Verification items for the finished model (mm, model axes). A direction names the side the tool comes from. Coordinates: 2 decimals unless noted, no trailing zeros. Loops run counter-clockwise (first coordinate to the right, second up) from the corner with the lowest first, then second, coordinate; pieces in that order, holes last. Notation, with made-up numbers: (36, 74) -> (61, 74) arc R31 ccw to (61, 103) -> close; hole circle Ø3 at (-22, 34). An arc over 180 degrees is marked (long way). Answer as a JSON object with one key per item and string values. Group by question number.
Q1. Gauge pin test, flat ends, axial feed: pin 1 Ø2 at (x, y) = (-21.5, -30.5) entering from -Z; pin 2 Ø1.1 at (x, y) = (-29.5, -30) entering from -Z; pin 3 Ø2 at (x, y) = (8, 35) entering from -Z; pin 4 Ø8 at (x, y) = (8.5, 27) entering from -Z. Record the tip position at first contact, or that the pin passes through.
Q2. Scan lines: L1, parallel to Y at x = 21.5, z = 6.25; L2, parallel to Y at x = 31, z = 4; L3, parallel to X at y = 31, z = 2. Record each from-to range of solid material in increasing order.
Q3. Cross-section at B-B on y = 10. Record the boundary of the cut face in (x, z).
Q4. Release check for a two-part mould opening along Y. For faces 1 (the flat face through (-30, 34.858, 8)), 2 (the flat face through (-26.56, -30.76, 11.35)), 3 (the flat face through (-28.03, 34.34, 1.48)) record: released by +Y, released by -Y, zero draft, split by the parting line, or undercut.
Q5. Set-up check for faces 4 (the flat face through (32, 2, 0)), 5 (the flat face through (-14.262, 34.872, 12.506)), 6 (the flat face through (-28.03, -28.22, 3.48)), 7 (the flat face through (4, 35, 5)), 8 (the flat face through (0, -31, 20)): record each of +Z, -Z, +X, -X, +Y, -Y from which the full face is reachable in a straight line by a thin tool's end or side.
Q6. Cross-section at C-C on x = 25.5. Record the boundary of the cut face in (y, z), and give its area (3 significant figures).
Q7. Cross-section at D-D on x = -30. Record the boundary of the cut face in (y, z), and give its area (3 significant figures).
Q8. Cross-section at A-A on z = 1. Record the boundary of the cut face in (x, y).
```python
from build123d import *

# Parameters (mm, degrees)
SKETCH2_W               = 70
SKETCH2_H               = 67.6
BOSS_EXTRUDE2_DEPTH     = 20
SKETCH3_W               = 49.211808989
SKETCH3_H               = 73.758147992
CUT_EXTRUDE1_DEPTH      = 5
SHELL1_T                = -2
CHAMFER1_SIZE           = 3
CHAMFER2_SIZE           = 3
CUT_EXTRUDE2_REACH      = 80.917
FILLET1_R               = 1
FILLET1_OF_MIRROR1_R    = 1
SKETCH6_W               = 4.489342342
SKETCH6_H               = 3.232194467
CUT_EXTRUDE3_DEPTH      = 1
MIRROR3_COPY_1_SKETCH_W = 4.489342342
MIRROR3_COPY_1_SKETCH_H = 3.232194467
MIRROR3_COPY_1_DEPTH    = 1


with BuildPart() as part:
    # Sketch2 → Boss-Extrude2 (new body)
    with BuildSketch(Plane.XY):
        with Locations((0.470659816, 2.057998975)):
            Rectangle(SKETCH2_W, SKETCH2_H)
    extrude(amount=BOSS_EXTRUDE2_DEPTH)

    # Sketch3 → Cut-Extrude1 (cut)
    with BuildSketch(Plane(origin=(0, 0, 0), x_dir=(-1, 0, 0), z_dir=(0, 0, -1))):
        with Locations((-3.250634913, 2.948650711)):
            Rectangle(SKETCH3_W, SKETCH3_H)
    extrude(amount=-CUT_EXTRUDE1_DEPTH, mode=Mode.SUBTRACT)

    # Shell1
    shell1_openings = [part.faces().sort_by_distance(p)[0] for p in [
        (0.470659816, 2.057998975, 20),
        (3.250634912, 2.057998975, 5),
        (-21.355269582, 2.057998975, 2.5),
        (27.856539407, 2.057998975, 2.5),
        (35.470659816, 2.057998975, 10),
        (-34.529340184, 2.057998975, 10),
    ]]
    offset(amount=SHELL1_T, openings=shell1_openings, kind=Kind.INTERSECTION)

    # Chamfer1
    chamfer1_edges = [part.edges().sort_by_distance(p)[0] for p in [
        (-27.942304883, -29.742001025, 2),
        (31.663599611, -29.742001025, 2),
        (-27.942304883, 33.857998975, 2),
        (31.663599611, 33.857998975, 2),
        (-27.942304883, -31.742001025, 0),
        (31.663599611, -31.742001025, 0),
        (31.663599611, 35.857998975, 0),
        (-27.942304883, 35.857998975, 0),
    ]]
    chamfer(chamfer1_edges, length=CHAMFER1_SIZE)

    # Chamfer2
    chamfer2_edges = [part.edges().sort_by_distance(p)[0] for p in [
        (35.470659816, -30.742001025, 20),
        (-34.529340184, -30.742001025, 20),
        (35.470659816, 34.857998975, 20),
        (-34.529340184, 34.857998975, 20),
    ]]
    chamfer(chamfer2_edges, length=CHAMFER2_SIZE)

    # Sketch5 → Cut-Extrude2 (cut, up to next)
    with BuildSketch(Plane(origin=(0, 35.857998975, 0), x_dir=(1, 0, 0), z_dir=(0, 1, 0)), mode=Mode.PRIVATE) as cut_extrude2_sk1:
        Polygon((-29.190337507, -15.412371153), (-16.14250414, -15.412371153), (-11.632506267, -8.443693022), (-24.680339633, -8.443693022), align=None)
    cut_extrude2_tool1 = extrude(cut_extrude2_sk1.sketch, amount=-CUT_EXTRUDE2_REACH, mode=Mode.PRIVATE) & part.part
    # Sketch5 → Cut-Extrude2 (cut, up to next)
    with BuildSketch(Plane(origin=(0, 35.857998975, 0), x_dir=(1, 0, 0), z_dir=(0, 1, 0)), mode=Mode.PRIVATE) as cut_extrude2_sk2:
        Polygon((-9.190337507, -15.412371153), (3.85749586, -15.412371153), (8.367493733, -8.443693022), (-4.680339633, -8.443693022), align=None)
    cut_extrude2_tool2 = extrude(cut_extrude2_sk2.sketch, amount=-CUT_EXTRUDE2_REACH, mode=Mode.PRIVATE) & part.part
    # Sketch5 → Cut-Extrude2 (cut, up to next)
    with BuildSketch(Plane(origin=(0, 35.857998975, 0), x_dir=(1, 0, 0), z_dir=(0, 1, 0)), mode=Mode.PRIVATE) as cut_extrude2_sk3:
        Polygon((10.809662493, -15.412371153), (23.85749586, -15.412371153), (28.367493733, -8.443693022), (15.319660367, -8.443693022), align=None)
    cut_extrude2_tool3 = extrude(cut_extrude2_sk3.sketch, amount=-CUT_EXTRUDE2_REACH, mode=Mode.PRIVATE) & part.part
    cut_extrude2_1 = cut_extrude2_tool1.solids().sort_by_distance((-20.411422, 35.857999, 11.928032))[0]
    add(cut_extrude2_1, mode=Mode.SUBTRACT)
    cut_extrude2_2 = cut_extrude2_tool2.solids().sort_by_distance((-0.411422, 35.857999, 11.928032))[0]
    add(cut_extrude2_2, mode=Mode.SUBTRACT)
    cut_extrude2_3 = cut_extrude2_tool3.solids().sort_by_distance((19.588578, 35.857999, 11.928032))[0]
    add(cut_extrude2_3, mode=Mode.SUBTRACT)
    cut_extrude2 = cut_extrude2_1 + cut_extrude2_2 + cut_extrude2_3  # Cut-Extrude2 as one shape, for the pattern or mirror that repeats it

    # Fillet1
    fillet1_edges = [part.edges().sort_by_distance(p)[0] for p in [
        (-16.14250414, 34.857998975, 15.412371153),
        (-11.632506267, 34.857998975, 8.443693022),
        (-24.680339633, 34.857998975, 8.443693022),
        (-29.190337507, 34.857998975, 15.412371153),
        (3.85749586, 34.857998975, 15.412371153),
        (8.367493733, 34.857998975, 8.443693022),
        (-4.680339633, 34.857998975, 8.443693022),
        (-9.190337507, 34.857998975, 15.412371153),
        (23.85749586, 34.857998975, 15.412371153),
        (28.367493733, 34.857998975, 8.443693022),
        (15.319660367, 34.857998975, 8.443693022),
        (10.809662493, 34.857998975, 15.412371153),
    ]]
    fillet(fillet1_edges, radius=FILLET1_R)

    # Mirror1: Cut-Extrude2 across plane
    add(cut_extrude2.mirror(Plane.ZX.offset(2.057998975)), mode=Mode.SUBTRACT)

    # Fillet1 of Mirror1
    fillet1_of_mirror1_edges = [part.edges().sort_by_distance(p)[0] for p in [
        (-16.14250414, -30.742001025, 15.412371153),
        (-11.632506267, -30.742001025, 8.443693022),
        (-24.680339633, -30.742001025, 8.443693022),
        (-29.190337507, -30.742001025, 15.412371153),
        (3.85749586, -30.742001025, 15.412371153),
        (8.367493733, -30.742001025, 8.443693022),
        (-4.680339633, -30.742001025, 8.443693022),
        (-9.190337507, -30.742001025, 15.412371153),
        (23.85749586, -30.742001025, 15.412371153),
        (28.367493733, -30.742001025, 8.443693022),
        (15.319660367, -30.742001025, 8.443693022),
        (10.809662493, -30.742001025, 15.412371153),
    ]]
    fillet(fillet1_of_mirror1_edges, radius=FILLET1_OF_MIRROR1_R)

    # Sketch6 → Cut-Extrude3 (cut)
    with BuildSketch(Plane(origin=(0, -29.742001025, 0), x_dir=(1, 0, 0), z_dir=(0, 1, 0))):
        with Locations((-29.492893563, -7.894775984)):
            Rectangle(SKETCH6_W, SKETCH6_H)
    cut_extrude3 = extrude(amount=-CUT_EXTRUDE3_DEPTH, mode=Mode.SUBTRACT)

    # Mirror2: Cut-Extrude3 across plane
    add(cut_extrude3.mirror(Plane.ZX.offset(2.057998975)), mode=Mode.SUBTRACT)

    # Mirror3: Cut-Extrude3 across plane
    add(cut_extrude3.mirror(Plane(origin=(0.470659816, 0, 0), x_dir=(0, 0, 1), z_dir=(1, 0, 0))), mode=Mode.SUBTRACT)

    # Mirror3 copy 1 sketch → Mirror3 copy 1 (cut)
    with BuildSketch(Plane(origin=(0.941319632, 33.857998975, 0), x_dir=(-1, 0, 0), z_dir=(0, -1, 0))):
        with Locations((-29.492893563, -7.894775984)):
            Rectangle(MIRROR3_COPY_1_SKETCH_W, MIRROR3_COPY_1_SKETCH_H)
    extrude(amount=-MIRROR3_COPY_1_DEPTH, mode=Mode.SUBTRACT)


solid = part.part
```
Computed values:
{
 "1": {"pin 1": "stops at z = 0.76", "pin 2": "stops at z = 0.71", "pin 3": "stops at z = 5", "pin 4": "passes through"},
 "2": {"L1": "y = -31.74 to -29.74, 33.86 to 35.86", "L2": "y = -31.74 to -28.74, 32.86 to 35.86", "L3": "x = -34.53 to -21.36, 27.86 to 35.47"},
 "3": {"outline": "(-34.53, 0) -> (-21.36, 0) -> (-21.36, 2) -> (-34.53, 2) -> close; (27.86, 0) -> (35.47, 0) -> (35.47, 2) -> (27.86, 2) -> close"},
 "4": {"face 1": "undercut", "face 2": "zero draft", "face 3": "released by +Y"},
 "5": {"face 4": "-Z, +X, -X, +Y, -Y", "face 5": "+Y, -Y", "face 6": "+Z, +X, -X", "face 7": "-Z, +Y, -Y", "face 8": "+Z, +X, -X, +Y, -Y"},
 "6": {"outline": "(-31.74, 5) -> (-29.74, 5) -> (-29.74, 8.44) -> (-31.74, 8.44) -> close; (-31.74, 12.87) -> (-29.74, 12.87) -> (-29.74, 20) -> (-31.74, 20) -> close; (33.86, 5) -> (35.86, 5) -> (35.86, 8.44) -> (33.86, 8.44) -> close; (33.86, 12.87) -> (35.86, 12.87) -> (35.86, 20) -> (33.86, 20) -> close", "area": "42.3 mm²"},
 "7": {"outline": "(-31.74, 3) -> (-28.74, 0) -> (32.86, 0) -> (35.86, 3) -> (35.86, 20) -> (33.86, 20) -> (33.86, 9.51) -> (34.86, 9.51) -> (34.86, 6.28) -> (33.86, 6.28) -> (33.86, 5) -> (30.86, 2) -> (-26.74, 2) -> (-29.74, 5) -> (-29.74, 6.28) -> (-30.74, 6.28) -> (-30.74, 9.51) -> (-29.74, 9.51) -> (-29.74, 20) -> (-31.74, 20) -> close", "area": "201 mm²"},
 "8": {"outline": "(-34.53, -29.74) -> (-21.36, -29.74) -> (-21.36, 33.86) -> (-34.53, 33.86) -> close; (27.86, -29.74) -> (35.47, -29.74) -> (35.47, 33.86) -> (27.86, 33.86) -> close"}
}
